The model under review builds one solid part; all positions refer to its coordinate system, in mm. A direction names the side the tool comes from. Round coordinates to 2 decimals unless told otherwise and drop trailing zeros. Order: outer loops, then holes, each group sorted by start corner. A loop starts at its lowest first (then second) coordinate and runs counter-clockwise, first axis right, second up.
1) Consider section B-B (z = 7.5). Give the boundary of the cut face in (x, y), then the cut area to 3 significant figures.
2) Mouldability with a two-part tool opening along X and no side actions: class faces 1 (the face through (110.995, 16.845, 7.742)), 2 (the face through (102.7, -2, 7.4)), 3 (the face through (-22, -23, 2)) as pulls with the +X half, pulls with the -X half, needs draft (parallel to the pull), parting line crosses it, or undercut.
3) Consider section A-A (x = 105.5). Give the boundary of the cut face in (y, z).
4) Clearance check with flat-ended pins moving along their axes: P1, Ø9, axis at x = 105, z = 7.5, coming from the +Y side; P2, Ø4.5, axis at x = 71, z = 4.5, coming from the -Y side; P3, Ø1.5, axis at x = 4, y = 10.5, coming from the +Z side. State where each tip first meets the part, or that it passes through.
5) Consider section D-D (y = -13.5). Give the boundary of the cut face in (x, z), then the cut area to 3 significant figures.
6) Consider section C-C (y = -22). Give the boundary of the cut face in (x, z), then the cut area to 3 significant figures.
7) Machinability: for faces 4 (the face through (18, -6, 5)), 5 (the face through (-10, -22, 2)), 6 (the face through (79, 20, 7)), 7 (the face through (103, 13.6, 5)), 8 (the face through (-23, 22, 2)), which of the approach directions +Z, -Z, +X, -X, +Y, -Y give a long, thin tool a straight path to every point of the face, cutting with its end or side? Answer none if there is none.
8) To check wall thickness, follow L1, parallel to Z at x = 105.5, y = 17.25; L2, parallel to Y at x = 99.5, z = 12.75; L3, parallel to Y at x = 90, z = 7. State the ranges of each line that lie inside material, in increasing order.
from build123d import *

# Parameters (mm, degrees)
ESQUISSE1_R                                        = 11
BOSS_EXTRU_1_DEPTH                                 = 15
CHAMBRAGE_POUR_VIS_T_TE_HEXAGONALE_M61_D           = 6.6
CHAMBRAGE_POUR_VIS_T_TE_HEXAGONALE_M61_DEPTH       = 18
CHAMBRAGE_POUR_VIS_T_TE_HEXAGONALE_M61_CBORE_D     = 11
CHAMBRAGE_POUR_VIS_T_TE_HEXAGONALE_M61_CBORE_DEPTH = 6.4
ENL_V_MAT_EXTRU_7_DEPTH                            = 91
TROU_TARAUD_M61_D                                  = 5
ENL_V_MAT_EXTRU_8_DEPTH                            = 6


with BuildPart() as part:
    # Esquisse1 → Boss.-Extru.1 (new body)
    with BuildSketch(Plane.XY):
        with BuildLine():
            Line((37, 30), (47, 20))
            Line((47, 20), (112, 20))
            Line((112, 20), (112, 2))
            Line((112, 2), (99.287087811, 2))
            ThreePointArc((99.287087811, 2), (80.5, 0), (99.287087811, -2))
            Line((99.287087811, -2), (112, -2))
            Line((112, -2), (112, -20))
            Line((112, -20), (47, -20))
            Line((47, -20), (37, -30))
            Line((37, -30), (-15, -30))
            Line((-15, -30), (-30, -15))
            Line((-30, -15), (-30, 15))
            Line((-30, 15), (-15, 30))
            Line((-15, 30), (37, 30))
        make_face()
        Circle(ESQUISSE1_R, mode=Mode.SUBTRACT)
        with BuildLine():
            Line((-8, 24), (8, 24))
            ThreePointArc((8, 24), (10, 22), (8, 20))
            Line((8, 20), (-8, 20))
            ThreePointArc((-8, 20), (-10, 22), (-8, 24))
        make_face(mode=Mode.SUBTRACT)
        with BuildLine():
            Line((-8, -24), (8, -24))
            ThreePointArc((8, -24), (10, -22), (8, -20))
            Line((8, -20), (-8, -20))
            ThreePointArc((-8, -20), (-10, -22), (-8, -24))
        make_face(mode=Mode.SUBTRACT)
    extrude(amount=BOSS_EXTRU_1_DEPTH)

    # Chambrage pour vis à tête hexagonale M61
    with Locations(Plane(origin=(0, 20, 0), x_dir=(-1, 0, 0), z_dir=(0, 1, 0))):
        with Locations((-105.5, 7.5)):
            CounterBoreHole(CHAMBRAGE_POUR_VIS_T_TE_HEXAGONALE_M61_D / 2, CHAMBRAGE_POUR_VIS_T_TE_HEXAGONALE_M61_CBORE_D / 2, CHAMBRAGE_POUR_VIS_T_TE_HEXAGONALE_M61_CBORE_DEPTH, depth=CHAMBRAGE_POUR_VIS_T_TE_HEXAGONALE_M61_DEPTH)

    # Esquisse4 → Enlèv. mat.-Extru.7 (cut, through all)
    with BuildSketch(Plane(origin=(0, 60, 0), x_dir=(1, 0, 0), z_dir=(0, 1, 0))):
        Polygon((47, -5), (-30, -5), (-30, -38.86865167), (80.86865167, -38.86865167), align=None)
    extrude(amount=-ENL_V_MAT_EXTRU_7_DEPTH, mode=Mode.SUBTRACT)

    # Trou taraudé M61 (through all)
    with Locations(Plane(origin=(0, -2, 0), x_dir=(1, 0, 0), z_dir=(0, 1, 0))):
        with Locations((105.5, -7.5)):
            Hole(TROU_TARAUD_M61_D / 2)

    # Esquisse7 → Enlèv. mat.-Extru.8 (cut, through all)
    with BuildSketch(Plane.XY.offset(5)):
        with BuildLine():
            Line((-24.3, 2), (-6.3, 2))
            ThreePointArc((-6.3, 2), (-4.3, 0), (-6.3, -2))
            Line((-6.3, -2), (-24.3, -2))
            ThreePointArc((-24.3, -2), (-26.3, 0), (-24.3, 2))
        make_face()
        with BuildLine():
            Line((8.8, 2), (30.8, 2))
            ThreePointArc((30.8, 2), (32.8, 0), (30.8, -2))
            Line((30.8, -2), (8.8, -2))
            ThreePointArc((8.8, -2), (6.8, 0), (8.8, 2))
        make_face()
    extrude(amount=-ENL_V_MAT_EXTRU_8_DEPTH, mode=Mode.SUBTRACT)


solid = part.part
Answer below:
1. outline: (49.5, -20) - (103, -20) - (103, -2) - (99.29, -2) arc R9.5 cw (long way) to (99.29, 2) - (102.2, 2) - (102.2, 13.6) - (100, 13.6) - (100, 20) - (49.5, 20) - close; (108, -20) - (112, -20) - (112, -2) - (108, -2) - close; (108.8, 2) - (112, 2) - (112, 20) - (111, 20) - (111, 13.6) - (108.8, 13.6) - close
1. area: 1,930 mm2
2. face 1: undercut
2. face 2: needs draft
2. face 3: pulls with the -X half
3. outline: (-20, 0) - (-2, 0) - (-2, 5) - (-20, 5) - close; (-20, 10) - (-2, 10) - (-2, 15) - (-20, 15) - close; (2, 0) - (20, 0) - (20, 2) - (13.6, 2) - (13.6, 4.2) - (2, 4.2) - close; (2, 10.8) - (13.6, 10.8) - (13.6, 13) - (20, 13) - (20, 15) - (2, 15) - close
4. P1: stops at y = 13.6
4. P2: stops at y = -20
4. P3: stops at z = 5
5. outline: (-30, 0) - (112, 0) - (112, 15) - (57, 15) - (47, 5) - (-30, 5) - close; hole circle Ø5 at (105.5, 7.5)
5. area: 1,290 mm2
6. outline: (-23, 0) - (-10, 0) - (-10, 5) - (-23, 5) - close; (10, 0) - (45, 0) - (45, 5) - (10, 5) - close
6. area: 240 mm2
7. face 4: +Z, -X, +Y, -Y
7. face 5: +Z, -Z
7. face 6: +Z, -Z, +X, +Y
7. face 7: +Y
7. face 8: +Z, -Z, -X, +Y
8. L1: z = 0 to 2, 13 to 15
8. L2: y = -20 to -2, 2 to 20
8. L3: y = -20 to -9.5, 9.5 to 20
